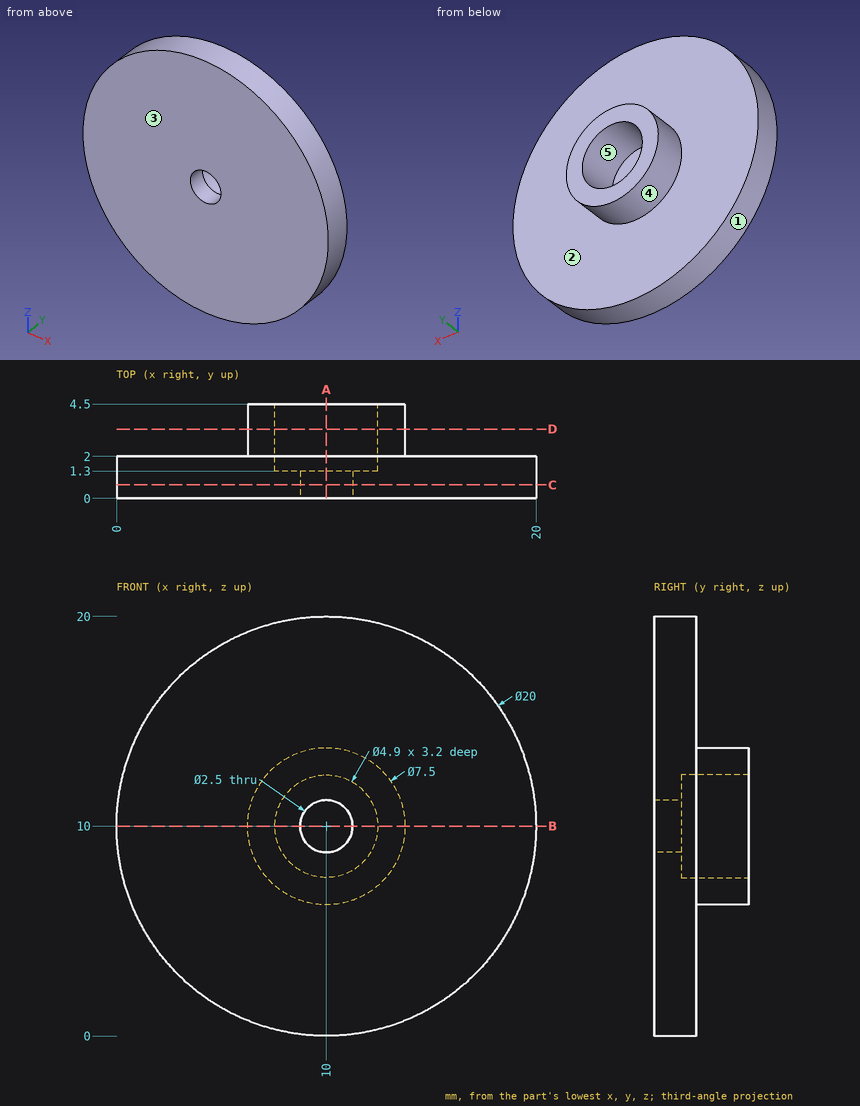
Geometry: see drawing. Coordinates: mm, zero at the bounding-box minimum. A direction names the side the tool comes from. Give positions to 0.01 mm unless a question says otherwise; leave off trailing zeros. Order: outer loops, then holes, each group sorted by start corner. A loop starts at its lowest first (then second) coordinate and runs counter-clockwise, first axis right, second up. Notation, with made-up numbers: (67, -10.5) -> (95, -10.5) arc R27 cw to (95, 11.5) -> close; hole circle Ø7 at (65, 51.25). An arc over 180 degrees is marked (long way). Write each question's results on one line, items separated by ' | '. Start each with the question number.
1) Section C-C (y = 0.65). Return loops of the section in (x, z).
2) Set-up query: the marked faces 1 and 2. Return all of +Z, -Z, +X, -X, +Y, -Y with unobstructed straight access to the full face (end or side cutting, diameter ignored); none if empty.
3) Line query: line 1 (X direction, y = 0.35, z = 10); line 2 (X direction, y = 3.6, z = 10); line 3 (Y direction, x = 6, z = 1.75). Output: solid intervals per line, ascending. Write a range as from..to.
4) Section B-B (z = 10). Return loops of the section in (x, y).
5) Section D-D (y = 3.3). Return loops of the section in (x, z), then the cut area to 3 significant figures.
6) Draft query along Z for the marked faces 3, 4 and 5. Return one class per face: pulls with the +Z half, pulls with the -Z half, needs draft (parallel to the pull), parting line crosses it, or undercut.
7) Section A-A (x = 10). Return loops of the section in (y, z), then the cut area to 3 significant figures.
8) First-contact query: pin 1 (4.5 mm diameter, centred on x = 10, z = 10, fed in from +Y). Flat tip, straight axial feed; report the tip coordinate or a pass-through.
Calculated:
1) outline: circle Ø20 at (10, 10); hole circle Ø2.5 at (10, 10)
2) face 1: +Y, -Y | face 2: +Y
3) line 1: 0..8.75, 11.25..20 | line 2: 6.25..7.55, 12.45..13.75 | line 3: 0..2
4) outline: (0, 0) -> (8.75, 0) -> (8.75, 1.3) -> (7.55, 1.3) -> (7.55, 4.5) -> (6.25, 4.5) -> (6.25, 2) -> (0, 2) -> close; (11.25, 0) -> (20, 0) -> (20, 2) -> (13.75, 2) -> (13.75, 4.5) -> (12.45, 4.5) -> (12.45, 1.3) -> (11.25, 1.3) -> close
5) outline: circle Ø7.5 at (10, 10); hole circle Ø4.9 at (10, 10) | area: 25.3 mm2
6) face 3: needs draft | face 4: parting line crosses it | face 5: undercut
7) outline: (0, 0) -> (2, 0) -> (2, 6.25) -> (4.5, 6.25) -> (4.5, 7.55) -> (1.3, 7.55) -> (1.3, 8.75) -> (0, 8.75) -> close; (0, 11.25) -> (1.3, 11.25) -> (1.3, 12.45) -> (4.5, 12.45) -> (4.5, 13.75) -> (2, 13.75) -> (2, 20) -> (0, 20) -> close | area: 39.8 mm2
8) pin 1: y = 1.3
